Autodesk Fusion 360 part; units mm, degrees
sketch "MASTER SKETCH" plane through (0, 0, 0) normal (0, 1, 0) x (1, 0, 0)
  line L0 (-20.1125, 7.8888) -> (9.6034, 8.2112)
  arc A0 (9.6034, 8.2112) -> (11.0867, 6.3443) centre (11.9278, 8.5352) ccw
  line L1 (11.0867, 6.3443) -> (11.0867, 5.2219)
  line L2 (11.0867, 5.2219) -> (21.1539, 5.2219)
  line L3 (21.1539, 5.2219) -> (21.1539, -4.9577)
  line L4 (21.1539, -4.9577) -> (11.0867, -4.9577)
  line L5 (11.0867, -4.9577) -> (11.0867, -5.8142)
  arc A1 (11.0867, -5.8142) -> (9.8311, -7.945) centre (11.8441, -7.6959) ccw
  line L6 (9.8311, -7.945) -> (-19.9558, -8.3433)
  arc A2 (-20.1125, 7.8888) -> (-19.9558, -8.3433) centre (-3.1266, -0.064) ccw
  line L7 (15.1779, 3.7868) -> (16.7624, 3.7868)
  line L8 (16.7624, 3.7868) -> (16.7624, 1.8338)
  line L9 (16.7624, 1.8338) -> (15.1779, 1.8338)
  line L10 (15.1779, 1.8338) -> (15.1779, 3.7868)
  line L11 (15.1779, -1.2246) -> (16.7624, -1.2246)
  line L12 (16.7624, -1.2246) -> (16.7624, -3.2144)
  line L13 (16.7624, -3.2144) -> (15.1779, -3.2144)
  line L14 (15.1779, -3.2144) -> (15.1779, -1.2246)
  circle A3 centre (-7.2793, 0.4193) radius 4.0763
extrude "Extrude1" add sketch "MASTER SKETCH" along normal blind 6.35 contours L0 A0 L1 L2 L3 L4 L5 A1 L6 A2 | L7 L8 L9 L10 | L11 L12 L13 L14 | A3 in component "BODY"
fillet "Fillet1" radius 3.175 4 edges at (-5.0623, 6.35, 8.1442) (-5.2545, 6.35, -8.05) (-5.0623, 0, 8.1442) (-5.2545, 0, -8.05) in component "BODY"
sketch "Sketch1" plane through (0, 6.35, 0) normal (0, 1, 0) x (-1, 0, 0) in component "BODY"
  line L0 (-21.1539, -5.1613) -> (21.2666, -4.7011)
  arc A0 (21.2666, -4.7011) -> (21.1696, 5.1842) centre (3.1266, 0.064) ccw
  line L1 (21.1696, 5.1842) -> (-21.1539, 4.6184)
  line L2 (-21.1539, 4.6184) -> (-21.1539, -5.1613)
  line L3 (-11.0867, -6.3443) -> (-11.0867, 5.8142)
  line L4 (-11.0867, 5.8142) -> (-21.1539, 5.8142)
  line L5 (-21.1539, 5.8142) -> (-21.1539, -6.3443)
  line L6 (-21.1539, -6.3443) -> (-11.0867, -6.3443)
extrude "Extrude2" cut sketch "Sketch1" against normal blind 1.27 contours L0 L1 L2 L3 L5 | L0 L3 L5 L6 | L1 L3 L4 L5 in component "BODY"
sketch "Sketch2" plane through (0, 0, 0) normal (0, -1, 0) x (1, 0, 0) in component "BODY"
  line L0 (-21.2666, -4.7011) -> (21.1539, -5.1613)
  line L1 (21.1539, -5.1613) -> (21.1539, 4.6184)
  line L2 (21.1539, 4.6184) -> (-21.1696, 5.1842)
  arc A0 (-21.1696, 5.1842) -> (-21.2666, -4.7011) centre (-3.1266, 0.064) ccw
  line L3 (11.0867, 5.8142) -> (11.0867, -6.3443)
  line L4 (11.0867, -6.3443) -> (21.1539, -6.3443)
  line L5 (21.1539, -6.3443) -> (21.1539, 5.8142)
  line L6 (21.1539, 5.8142) -> (11.0867, 5.8142)
extrude "Extrude3" cut sketch "Sketch2" against normal blind 1.27 contours L0 L1 L2 L3 L5 | L0 L3 L4 L5 | L2 L3 L5 L6 in component "BODY"
sketch "Sketch3" plane through (0, 5.08, 0) normal (0, 1, 0) x (-1, 0, 0) in component "BODY"
  line L0 (-21.1539, -5.2219) -> (-11.0867, -5.2219)
  line L1 (-11.0867, -5.2219) -> (-11.0867, 4.9577)
  line L2 (-11.0867, 4.9577) -> (-21.1539, 4.9577)
  line L3 (-21.1539, 4.9577) -> (-21.1539, -5.2219)
  line L4 (-15.8492, -3.9519) -> (-17.3439, -3.9519)
  line L5 (-17.3439, -3.9519) -> (-17.3439, -2.0273)
  line L6 (-17.3439, -2.0273) -> (-15.8492, -2.0273)
  line L7 (-15.8492, -2.0273) -> (-15.8492, -3.9519)
  line L8 (-15.8492, 1.7827) -> (-17.3439, 1.7827)
  line L9 (-17.3439, 1.7827) -> (-17.3439, 3.6681)
  line L10 (-17.3439, 3.6681) -> (-15.8492, 3.6681)
  line L11 (-15.8492, 3.6681) -> (-15.8492, 1.7827)
  dimension "d8" = 3.81
  dimension "d9" = 7.62
  dimension "d10" = 4.7625
  dimension "d11" = 4.7625
  dimension "d12" = 3.81
  dimension "d13" = 3.81
  dimension "d14" = 3.81
  dimension "d15" = 1.27
  dimension "d16" = 6.985
sketch "Sketch4" plane through (21.1539, 0, 0) normal (1, 0, 0) x (0, 0, -1) in component "BODY"
  line L0 (-4.9577, 1.27) -> (5.2219, 1.27)
  line L1 (5.2219, 1.27) -> (5.2219, 5.08)
  line L2 (5.2219, 5.08) -> (-4.9577, 5.08)
  line L3 (-4.9577, 5.08) -> (-4.9577, 1.27)
  line L4 (-4.9577, 5.08) -> (-4.9577, 4.445)
  line L5 (-4.9577, 4.445) -> (-4.3227, 4.445)
  line L6 (5.2219, 5.08) -> (5.2219, 4.445)
  line L7 (5.2219, 4.445) -> (4.5869, 4.445)
  line L8 (4.5869, 4.445) -> (-4.3227, 4.445)
  line L9 (-4.3227, 4.445) -> (-4.3227, 2.413)
  line L10 (-4.3227, 2.413) -> (4.5869, 2.413)
  line L11 (4.5869, 2.413) -> (4.5869, 4.445)
  dimension "d17" = 0.635
  dimension "d18" = 0.635
  dimension "d19" = 0.635
  dimension "d20" = 0.635
  dimension "d21" = 2.032
extrude "Extrude4" cut sketch "Sketch4" against normal blind 11.43 contours L8 L9 L10 L11 in component "BODY"
sketch "Sketch5" plane through (0, 2.413, 0) normal (0, 1, 0) x (-1, 0, 0) in component "BODY"
extrude "Extrude5" cut sketch "Sketch3" against normal blind 1.778 contours L4 L5 L6 L7 | L8 L9 L10 L11 in component "BODY"
sketch "Sketch6" plane through (0, 6.35, 0) normal (0, 1, 0) x (-1, 0, 0) in component "BODY"
  line L0 (-11.0867, 4.753) -> (-11.0867, -5.0521)
  line L1 (-11.0867, -5.0521) -> (21.2666, -4.7011)
  arc A0 (21.2666, -4.7011) -> (21.1696, 5.1842) centre (3.1266, 0.064) ccw
  line L2 (21.1696, 5.1842) -> (-11.0867, 4.753)
  circle A1 centre (7.1973, -0.1496) radius 4.0638
extrude "Extrude6" add sketch "Sketch6" along normal blind 0.635 contours A1 in component "BODY"
sketch "Sketch7" plane through (0, 0, 0) normal (0, -1, 0) x (1, 0, 0) in component "BODY"
  line L0 (11.0867, -5.0521) -> (11.0867, 4.753)
  line L1 (11.0867, 4.753) -> (-21.1696, 5.1842)
  arc A0 (-21.1696, 5.1842) -> (-21.2666, -4.7011) centre (-3.1266, 0.064) ccw
  line L2 (-21.2666, -4.7011) -> (11.0867, -5.0521)
  circle A1 centre (-7.1973, 0) radius 4.0638
extrude "Extrude7" add sketch "Sketch7" along normal blind 0.635 contours A1 in component "BODY"
fillet "Fillet2" radius 0.635 2 edges at (-10.9861, -0.635, -1.4695) (-3.4085, 6.985, -1.6191) 1 faces at (-8.4257, -0.635, 1.6844) in component "BODY"
sketch "Sketch8" plane through (0, 5.08, 0) normal (0, 1, 0) x (-1, 0, 0) in component "BODY"
  line L0 (-17.3439, -3.9519) -> (-17.3439, -2.0273)
  line L1 (-17.3439, -2.0273) -> (-15.8492, -2.0273)
  line L2 (-15.8492, -2.0273) -> (-15.8492, -3.9519)
  line L3 (-15.8492, -3.9519) -> (-17.3439, -3.9519)
  line L4 (-17.3439, 1.7827) -> (-17.3439, 3.6681)
  line L5 (-17.3439, 3.6681) -> (-15.8492, 3.6681)
  line L6 (-15.8492, 3.6681) -> (-15.8492, 1.7827)
  line L7 (-15.8492, 1.7827) -> (-17.3439, 1.7827)
  line L8 (-21.1539, -5.2219) -> (-11.0867, -5.2219)
  line L9 (-11.0867, -5.2219) -> (-11.0867, 4.9577)
  line L10 (-11.0867, 4.9577) -> (-21.1539, 4.9577)
  line L11 (-21.1539, 4.9577) -> (-21.1539, -5.2219)
  line L12 (-15.8492, -3.9519) -> (-17.3439, -3.9519)
  line L13 (-17.3439, -3.9519) -> (-17.3439, -2.0273)
  line L14 (-17.3439, -2.0273) -> (-15.8492, -2.0273)
  line L15 (-15.8492, -2.0273) -> (-15.8492, -3.9519)
  line L16 (-15.8492, 1.7827) -> (-17.3439, 1.7827)
  line L17 (-17.3439, 1.7827) -> (-17.3439, 3.6681)
  line L18 (-17.3439, 3.6681) -> (-15.8492, 3.6681)
  line L19 (-15.8492, 3.6681) -> (-15.8492, 1.7827)
extrude "Extrude8" cut sketch "Sketch8" against normal blind 5.842 contours L0 L1 L2 L3 L12 L13 L14 L15 | L4 L5 L6 L7 L16 L17 L18 L19 in component "BODY"
component "BODY" placed x (1, 0, 0) y (0, 1, 0) z (0, 0, 1) at (0, 0, 0)
Geometry check sheet. Reference: the model listing, model coordinates, mm. A direction names the side the tool comes from. Give positions to 0.01 mm unless a question says otherwise; leave off trailing zeros. Loops run counter-clockwise (first coordinate to the right, second up) from the corner with the lowest first, then second, coordinate; pieces in that order, holes last.
(1) Set-up check for faces 5 (the cylindrical face through (-4.88, 0.905, -7.099)), 6 (the flat face through (16, 1.27, 0)), 7 (the cylindrical face through (-5.237, 0.905, 7.192)), 8 (the flat face through (17, 2, -2.027)), 9 (the flat face through (16, 3, 4.958)): record each of +Z, -Z, +X, -X, +Y, -Y from which the full face is reachable in a straight line by a thin tool's end or side.
From the geometry:
face 5: -Z, -X, -Y
face 6: +Z, -Z, +X, -Y
face 7: +Z, +X, -Y
face 8: +Y, -Y
face 9: +Z, +X, +Y, -Y
(2) Thickness scan on L1, parallel to Y at x = 17.5, z = -3.5 (3 decimals); L2, parallel to Y at x = -15, z = 2.5; L3, parallel to Z at x = 12.5, y = 2.5. Record the ranges inside material, lowest first.
From the geometry:
L1: y = 1.27 to 2.413, 4.445 to 5.08
L2: y = 0 to 6.35
L3: z = -5.22 to -4.59, 4.32 to 4.96
(3) Section check A-A on x = 13. Record the cut outline in (y, z) (3 decimals), then the cut area to 3 significant figures.
From the geometry:
outline: (1.27, -5.222) - (5.08, -5.222) - (5.08, 4.958) - (1.27, 4.958) - close; hole (2.413, -4.587) - (4.445, -4.587) - (4.445, 4.323) - (2.413, 4.323) - close
area: 20.7 mm2
(4) Depth check by flat-ended pin: pin 1 Ø1.5 at (x, y) = (-16, 1.5) entering from -Z; pin 2 Ø1.1 at (x, y) = (16, 2.5) entering from +Z; pin 3 Ø1.5 at (x, y) = (-8.5, 4.5) entering from -Z. Enter the tip coordinate at first touch or a pass-through.
From the geometry:
pin 1: stops at z = -7.8
pin 2: stops at z = 4.96
pin 3: stops at z = -7.96
(5) Release check for a two-part mould opening along Y. For faces 1 (the flat face through (9.724, 3, 0)), 2 (the flat face through (16, 2.413, 0)), 3 (the flat face through (17, 2, 1.783)), 4 (the flat face through (-2, 0, 0)) record: released by +Y, released by -Y, zero draft, split by the parting line, or undercut.
From the geometry:
face 1: undercut
face 2: undercut
face 3: zero draft
face 4: released by -Y
(6) Section check B-B on y = 2. Record the cut outline in (x, z), then the cut area to 3 significant figures.
From the geometry:
outline: (-20.22, -7.66) - (9.65, -7.99) arc R2.35 cw to (11.09, -6.34) - (11.09, -5.22) - (21.15, -5.22) - (21.15, 4.96) - (11.09, 4.96) - (11.09, 5.81) arc R2.03 cw to (9.82, 7.72) - (-20.06, 8.12) arc R18.76 ccw to start; hole (15.85, -3.95) - (17.34, -3.95) - (17.34, -2.03) - (15.85, -2.03) - close; hole (15.85, 1.78) - (17.34, 1.78) - (17.34, 3.67) - (15.85, 3.67) - close
area: 604 mm2
